Job drawing, mm, ordinate dimensions from the low corner. One solid piece. Coordinates: 2 decimals unless noted, no trailing zeros. Write each loop counter-clockwise with the first axis right and the second up, starting at its lowest first coordinate (ties: lowest second). Pieces come first, ordered by that corner, then holes. Notation, with made-up numbers: (73, 11) -> (112, 11) arc R13 ccw to (112, 21) -> close; hole circle Ø2 at (28.25, 89.5). An arc over 180 degrees is marked (long way). Answer as a JSON object with one key per item and string values. Group by question number.
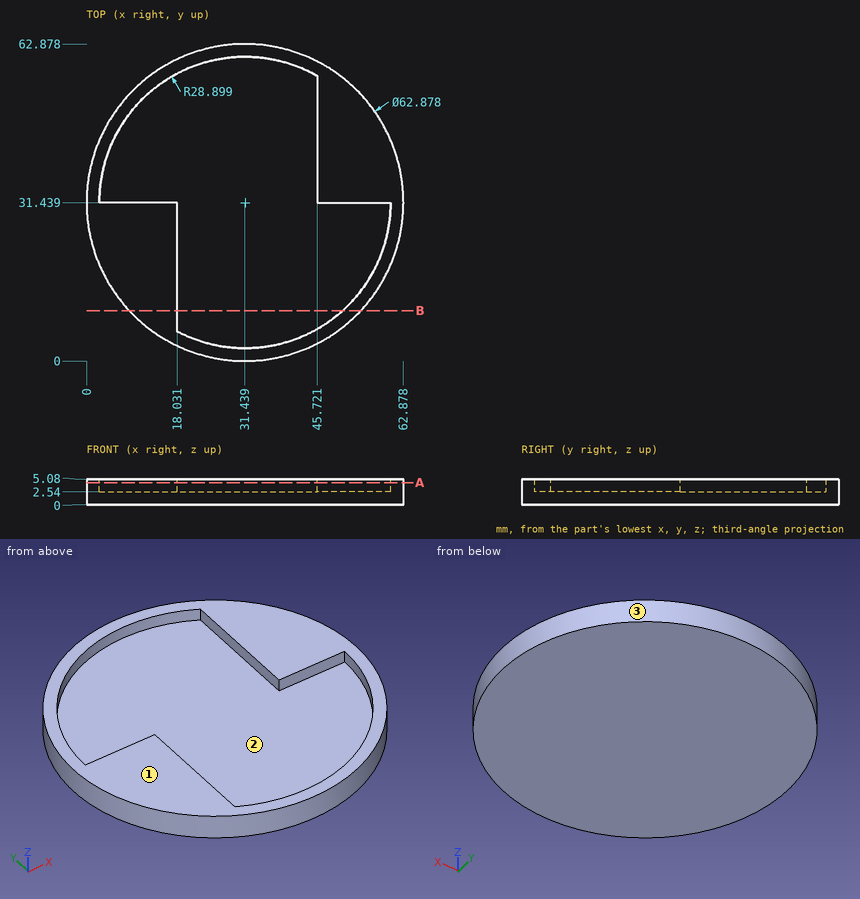
(1) Wall check: probe 1 along Z at (x, y) = (10, 31.5); probe 2 along X at (y, z) = (53, 3.5) (1 decimal); probe 3 along X at (y, z) = (35.5, 4.1) (1 decimal). Give the ranges that are in metal, low to high.
(2) Pull direction X, two halves, no side cores. Call the marked faces 1, 2 and 3: released by +X, released by -X, zero draft, split by the parting line, or undercut.
(3) Pin check, flat tips, straight feed: pin 1 (2 mm diameter, centred on y = 36.5, z = 3, fed in from -X); pin 2 (3 mm diameter, centred on x = 7, z = 4, fed in from +Y); pin 3 (1.3 mm diameter, centred on x = 52, z = 4.5, fed in from -Y). Stop position of each tip, or through.
(4) Cut at B-B on y = 10. List the corners of the cut face in (x, z) (1 decimal), plus the area to 3 significant figures.
(5) Cut at A-A on z = 4.35. List the corners of the cut face in (x, y), plus the area to 4 significant figures.
Results found:
{
 "1": {"probe 1": "z = 0 to 2.54", "probe 2": "x = 8.6 to 12.2, 45.7 to 54.3", "probe 3": "x = 0.3 to 2.8, 45.7 to 62.6"},
 "2": {"face 1": "zero draft", "face 2": "undercut", "face 3": "split by the parting line"},
 "3": {"pin 1": "stops at x = 0.26", "pin 2": "stops at y = 52.94", "pin 3": "stops at y = 7.11"},
 "4": {"outline": "(8.4, 0) -> (54.4, 0) -> (54.4, 5.1) -> (50.8, 5.1) -> (50.8, 2.5) -> (18, 2.5) -> (18, 5.1) -> (8.4, 5.1) -> close", "area": "150 mm²"},
 "5": {"outline": "circle Ø62.88 at (31.44, 31.44); hole (2.54, 31.44) -> (18.03, 31.44) -> (18.03, 5.84) arc R28.9 ccw to (60.34, 31.44) -> (45.72, 31.44) -> (45.72, 56.56) arc R28.9 ccw to start", "area": "1,025 mm²"}
}
